Autodesk Inventor part; units mm, degrees
ref_plane "YZ Plane" through (0, 0, 0) normal (1, 0, 0) x (0, 1, 0)
ref_plane "XZ Plane" through (0, 0, 0) normal (0, 1, 0) x (-1, 0, 0)
ref_plane "XY Plane" through (0, 0, 0) normal (0, 0, 1) x (1, 0, 0)
sketch "Sketch1" plane through (0, 0, 0) normal (0, 1, 0) x (-1, 0, 0)
  line L0 (-27.3558, 45.72) -> (27.3558, 45.72)
  line L1 (27.3558, 45.72) -> (27.3558, -45.72)
  line L2 (27.3558, -45.72) -> (-27.3558, -45.72)
  line L3 (-27.3558, -45.72) -> (-27.3558, 45.72)
  line L4 (-27.3558, 45.72) -> (27.3558, -45.72) construction
  line L5 (27.3558, 45.72) -> (-27.3558, -45.72) construction
  point P0 (0, 0)
  dimension "d0" = 54.7116
  dimension "d1" = 91.44
extrude "Extrusion1" add sketch "Sketch1" along normal blind 2.794
fillet "Fillet1" radius 3.175 4 edges at (-27.3558, 1.397, 45.72) (27.3558, 1.397, 45.72) (27.3558, 1.397, -45.72) (-27.3558, 1.397, -45.72)
sketch "Sketch2" plane through (0, 2.794, 0) normal (0, 1, 0) x (1, 0, 0)
  circle A0 centre (-6.3442, 0) radius 6.223
  circle A1 centre (-12.7676, 7.75) radius 1.5
  circle A2 centre (14.0792, 7.75) radius 1.5
  circle A3 centre (0.6558, 15.5) radius 1.5
  circle A4 centre (0.6558, -15.5) radius 1.5
  circle A5 centre (14.0792, -7.75) radius 1.5
  circle A6 centre (-12.7676, -7.75) radius 1.5
  line L0 (-27.3558, -45.72) -> (-27.3558, 45.72)
  line L1 (-27.3558, 45.72) -> (27.3558, 45.72)
  line L2 (27.3558, 45.72) -> (27.3558, -45.72)
  line L3 (27.3558, -45.72) -> (-27.3558, -45.72)
  circle A7 centre (0, 0) radius 18.415
  dimension "d5" = 36.83
extrude "Extrusion2" cut sketch "Sketch2" against normal blind 2.794 contours A0 | A1 | A2 | A3 | A4 | A5 | A6 | A7
sketch "Sketch3" plane through (0, 0, 0) normal (0, -1, 0) x (1, 0, 0)
  arc A0 (-39.5942, -30.48) -> (-36.5942, -30.48) centre (-38.0942, -30.48) ccw
  line L0 (-36.5942, -30.48) -> (-36.5942, -5.08)
  arc A1 (-36.5942, -5.08) -> (-39.5942, -5.08) centre (-38.0942, -5.08) ccw
  line L1 (-39.5942, -5.08) -> (-39.5942, -30.48)
  arc A2 (-39.5942, 5.08) -> (-36.5942, 5.08) centre (-38.0942, 5.08) ccw
  line L2 (-36.5942, 5.08) -> (-36.5942, 30.48)
  arc A3 (-36.5942, 30.48) -> (-39.5942, 30.48) centre (-38.0942, 30.48) ccw
  line L3 (-39.5942, 30.48) -> (-39.5942, 5.08)
  circle A4 centre (9.1558, -15.5) radius 1.5
  circle A5 centre (-21.8442, -15.5) radius 1.5
  circle A6 centre (9.1558, 15.5) radius 1.5
  circle A7 centre (-21.8442, 15.5) radius 1.5
  circle A8 centre (-6.3442, 0) radius 11
  line L4 (-10.7442, -50.8) -> (-20.9042, -50.8)
  line L5 (-20.9042, -50.8) -> (-20.9042, -45.72)
  line L6 (-20.9042, -45.72) -> (-31.0642, -45.72)
  line L7 (-31.0642, -45.72) -> (-31.0642, -50.8)
  line L8 (-31.0642, -50.8) -> (-41.2242, -50.8)
  line L9 (-41.2242, -50.8) -> (-41.2242, -45.72)
  line L10 (-41.2242, -45.72) -> (-46.3042, -45.72)
  line L11 (-46.3042, -45.72) -> (-46.3042, 45.72)
  line L12 (-46.3042, 45.72) -> (-41.2242, 45.72)
  line L13 (-41.2242, 45.72) -> (-41.2242, 50.8)
  line L14 (-41.2242, 50.8) -> (-31.0642, 50.8)
  line L15 (-31.0642, 50.8) -> (-31.0642, 45.72)
  line L16 (-31.0642, 45.72) -> (-20.9042, 45.72)
  line L17 (-20.9042, 45.72) -> (-20.9042, 50.8)
  line L18 (-20.9042, 50.8) -> (-10.7442, 50.8)
  line L19 (-10.7442, 50.8) -> (-10.7442, 45.72)
  line L20 (-10.7442, 45.72) -> (-0.5842, 45.72)
  line L21 (-0.5842, 45.72) -> (-0.5842, 50.8)
  line L22 (-0.5842, 50.8) -> (9.5758, 50.8)
  line L23 (9.5758, 50.8) -> (9.5758, 45.72)
  line L24 (9.5758, 45.72) -> (14.6558, 45.72)
  line L25 (14.6558, 45.72) -> (14.6558, -45.72)
  line L26 (14.6558, -45.72) -> (9.5758, -45.72)
  line L27 (9.5758, -45.72) -> (9.5758, -50.8)
  line L28 (9.5758, -50.8) -> (-0.5842, -50.8)
  line L29 (-0.5842, -50.8) -> (-0.5842, -45.72)
  line L30 (-0.5842, -45.72) -> (-10.7442, -45.72)
  line L31 (-10.7442, -45.72) -> (-10.7442, -50.8)
  point P0 (0, 0)
extrude "Extrusion3" cut sketch "Sketch3" against normal blind 2.794 contours A4 | A5 | A6 | A7
properties part number "MotorMountDC" material "Polycarbonate, Smoke"
Geometry check sheet. Reference: the model listing, model coordinates, mm. A direction names the side the tool comes from. Round coordinates to 2 decimals unless told otherwise and drop trailing zeros. Order: outer loops, then holes, each group sorted by start corner. A loop starts at its lowest first (then second) coordinate and runs counter-clockwise, first axis right, second up. Notation, with made-up numbers: (-5.5, 64.25) - (28.5, 64.25) arc R33 cw to (28.5, 96.25) - close; hole circle Ø1 at (11, 75). An arc over 180 degrees is marked (long way). Use a Markdown table: item, result. Add a question column.
(1) Sectioned sample at B-B, the plane z = 0. Enter the section's corners in (x, y) (3 decimals).
(2) Release check for a two-part mould opening along Z. For faces 3 (the cylindrical face through (-23.343, 1.377, -15.434)), 4 (the flat face through (-27.356, 1, 1)), 5 (the cylindrical face through (26.45, 1.417, -44.765)) record: pulls with the +Z half, pulls with the -Z half, needs draft (parallel to the pull), parting line crosses it, or undercut.
(3) Tool access check on faces 1 (the cylindrical face through (26.401, 1.417, 44.815)), 2 (the cylindrical face through (18.413, 1.417, 0.247)). Record the directions out of +Z, -Z, +X, -X, +Y, -Y that give a thin tool (end or side, any length) a straight path to the whole face; none if there is none.
(4) Material ranges on line 1 along X through (y, z) = (0.7, 0) (3 decimals); line 2 along Z through (x, y) = (0, 1.9) (3 decimals); line 3 along X through (y, z) = (0.6, -16), recorded low to high. Write a range as [from, to].
(5) Sectioned sample at C-C, the plane y = 2. Count the separate pieces of the cut face and the enclosed holes in it, and give its area (3 significant figures).
(6) Sectioned sample at A-A, the plane x = 0. Enter the section's corners in (y, z) (3 decimals), and give its area (3 significant figures).
Answers below:
| question | item | result |
|---|---|---|
| 1 | outline | (-27.356, 0) - (-18.415, 0) - (-18.415, 2.794) - (-27.356, 2.794) - close; (18.415, 0) - (27.356, 0) - (27.356, 2.794) - (18.415, 2.794) - close |
| 2 | face 3 | undercut |
| 2 | face 4 | needs draft |
| 2 | face 5 | pulls with the -Z half |
| 3 | face 1 | +Z, +X, +Y, -Y |
| 3 | face 2 | +Y, -Y |
| 4 | line 1 | [-27.356, -18.415], [18.415, 27.356] |
| 4 | line 2 | [-45.72, -18.415], [18.415, 45.72] |
| 4 | line 3 | [-27.36, -23.26], [-20.43, -9.12], [10.57, 27.36] |
| 5 | separate pieces | 1 |
| 5 | enclosed holes | 3 |
| 5 | area | 3,910 mm² |
| 6 | outline | (0, -45.72) - (2.794, -45.72) - (2.794, -18.415) - (0, -18.415) - close; (0, 18.415) - (2.794, 18.415) - (2.794, 45.72) - (0, 45.72) - close |
| 6 | area | 153 mm² |
